from build123d import *

# Parameters (mm, degrees)
BOSS_EXTRUDE1_DEPTH = 49
SKETCH7_W           = 31.1
SKETCH7_H           = 22
CUT_EXTRUDE5_DEPTH  = 3
SKETCH8_R           = 2.5
CUT_EXTRUDE6_DEPTH  = 3


with BuildPart() as part:
    # Sketch1 → Boss-Extrude1 (new body)
    with BuildSketch(Plane(origin=(0, 0, 0), x_dir=(0, 0, -1), z_dir=(1, 0, 0))):
        Polygon((-38, 0), (0, 0), (0, 23), (-3, 23), (-3, 3), (-38, 3), align=None)
    extrude(amount=BOSS_EXTRUDE1_DEPTH)

    # Sketch7 → Cut-Extrude5 (cut)
    with BuildSketch(Plane(origin=(0, 3, 0), x_dir=(1, 0, 0), z_dir=(0, 1, 0))):
        with Locations((23.55, -20)):
            Rectangle(SKETCH7_W, SKETCH7_H)
    extrude(amount=-CUT_EXTRUDE5_DEPTH, mode=Mode.SUBTRACT)

    # Sketch8 → Cut-Extrude6 (cut)
    with BuildSketch(Plane.XY.offset(3)):
        with Locations((14.5, 13)):
            Circle(SKETCH8_R)
        with Locations((34.5, 13)):
            Circle(SKETCH8_R)
    extrude(amount=-CUT_EXTRUDE6_DEPTH, mode=Mode.SUBTRACT)


solid = part.part
Check sheet for the modelled part. Datum: model origin and axes. Units: mm. A direction names the side the tool comes from. Round coordinates to 2 decimals unless told otherwise and drop trailing zeros. Loops run counter-clockwise (first coordinate to the right, second up) from the corner with the lowest first, then second, coordinate; pieces in that order, holes last. Notation, with made-up numbers: (32.25, 83) -> (78.25, 83) arc R18 cw to (78.25, 110) -> close; hole circle Ø3 at (10, -17.75). An arc over 180 degrees is marked (long way). Put each result on its own line as item: value. Start each with the question number.
1. Section check C-C (y = 1.5). Enter the section's corners in (x, z), plus the area to 3 significant figures.
2. Access from +Z, -Z, +X, -X, +Y, -Y to the whole of each face (thin tool, end or side, straight path). Record for faces 5 (the face through (24, 23, 1)), 6 (the face through (24, 13, 3)), 7 (the face through (23, 2, 9)).
3. Scan lines: probe 1 along X at (y, z) = (2.75, 17.5); probe 2 along Y at (x, z) = (34.5, 2.3); probe 3 along Z at (x, y) = (38.5, 19.5). Record each from-to range of solid material in increasing order.
4. Section check A-A (x = 16). Enter the section's corners in (y, z).
5. Section check D-D (x = 6.5). Enter the section's corners in (y, z).
6. Gauge pin test, flat ends, axial feed: pin 1 (2 mm diameter, centred on x = 42.5, y = 11.5, fed in from +Z); pin 2 (12 mm diameter, centred on y = 13.5, z = 17.5, fed in from -X). Record the tip position at first contact, or that the pin passes through.
7. Draft check along X on faces 1 (the face through (0, 2, 12)), 2 (the face through (23, 2, 31)), 3 (the face through (8, 2, 20)), 4 (the face through (24.2, 3, 8.6)). Enter one of: +X half, -X half, draft (parallel to the pull), parting line (faces both ways), or undercut.
8. Section check B-B (y = 13). Enter the section's corners in (x, z), plus the area to 3 significant figures.
Findings:
1. outline: (0, 0) -> (49, 0) -> (49, 38) -> (0, 38) -> close; hole (8, 9) -> (39.1, 9) -> (39.1, 31) -> (8, 31) -> close
1. area: 1,180 mm^2
2. face 5: +Z, -Z, +X, -X, +Y
2. face 6: +Z, +X, -X, +Y
2. face 7: +Y, -Y
3. probe 1: x = 0 to 8, 39.1 to 49
3. probe 2: y = 0 to 10.5, 15.5 to 23
3. probe 3: z = 0 to 3
4. outline: (0, 0) -> (11, 0) -> (11, 3) -> (3, 3) -> (3, 9) -> (0, 9) -> close; (0, 31) -> (3, 31) -> (3, 38) -> (0, 38) -> close; (15, 0) -> (23, 0) -> (23, 3) -> (15, 3) -> close
5. outline: (0, 0) -> (23, 0) -> (23, 3) -> (3, 3) -> (3, 38) -> (0, 38) -> close
6. pin 1: stops at z = 3
6. pin 2: passes through
7. face 1: -X half
7. face 2: undercut
7. face 3: undercut
7. face 4: draft
8. outline: (0, 0) -> (12, 0) -> (12, 3) -> (0, 3) -> close; (17, 0) -> (32, 0) -> (32, 3) -> (17, 3) -> close; (37, 0) -> (49, 0) -> (49, 3) -> (37, 3) -> close
8. area: 117 mm^2
